Verification items for the finished model (mm, model axes). A direction names the side the tool comes from. Coordinates: 2 decimals unless noted, no trailing zeros. Loops run counter-clockwise (first coordinate to the right, second up) from the corner with the lowest first, then second, coordinate; pieces in that order, holes last.
Q1. Access from +Z, -Z, +X, -X, +Y, -Y to the whole of each face (thin tool, end or side, straight path). Record for faces 1 (the face through (-7.493, 0.33, 29.249)), 2 (the face through (37.497, -16.228, 22.283)), 3 (the face through (-1.409, -17.325, 10.295)).
Q2. Sectioned sample at A-A (x = 0). Enter the section's corners in (y, z), then the cut area to 3 significant figures.
Q3. Sectioned sample at B-B (z = 20.5). Enter the section's corners in (x, y).
Q4. Sectioned sample at C-C (x = 33.5). Enter the section's corners in (y, z), then the cut area to 3 significant figures.
Q5. Material ranges on probe 1 along Y at (x, z) = (-6, 24); probe 2 along Z at (x, y) = (-26.5, -8); probe 3 along Y at (x, z) = (-8, 7.5), recorded low to high.
Q6. Go/stop test with flat-tipped pins: P1, Ø10, axis at x = 9, y = 7, coming from the -Z side; P2, Ø1, axis at y = 9, z = 6, coming from the +X side; P3, Ø12, axis at x = 8.5, y = 1, coming from the -Z side; P4, Ø12, axis at x = -11.5, y = -11, coming from the -Z side. Record where each tip stops, or that it passes through.
```python
from build123d import *

# Parameters (mm, degrees)
BOSS_EXTRUDE1_DEPTH      = 27.77
FILLET1_START            = -44
FILLET1_DEPTH            = 88
FILLET2_R                = 3
SKETCH3_R                = 7.5
BOSS_EXTRUDE2_DEPTH      = 3
BOSS_EXTRUDE3_DEPTH      = 2
BOSS_EXTRUDE3_DEPTH_BACK = 3
SKETCH4_R                = 6.5


with BuildPart() as part:
    # Sketch2 → Boss-Extrude1 (new body)
    with BuildSketch(Plane.XY):
        with BuildLine():
            Line((-37.65, 16.64), (37.65, 16.64))
            ThreePointArc((37.65, 16.64), (42.65, 0), (37.65, -16.64))
            Line((37.65, -16.64), (-37.65, -16.64))
            ThreePointArc((-37.65, -16.64), (-42.65, 0), (-37.65, 16.64))
        make_face()
    extrude(amount=BOSS_EXTRUDE1_DEPTH)

    # Fillet1: read off the stored shape, not the designer's step
    # Fillet1 outline → Fillet1 (cut)
    with BuildSketch(Plane.YZ.offset(FILLET1_START)):
        with BuildLine():
            Line((16.64, 0), (16.64, 16.64))
            ThreePointArc((16.64, 16.64), (11.766256851, 4.873743173), (3.4e-08, 0))
            Line((3.4e-08, 0), (16.64, 0))
        make_face()
        with BuildLine():
            Line((-16.64, 0), (3.4e-08, 0))
            ThreePointArc((3.4e-08, 0), (-11.766256827, 4.873743149), (-16.64, 16.64))
            Line((-16.64, 16.64), (-16.64, 0))
        make_face()
    extrude(amount=FILLET1_DEPTH, mode=Mode.SUBTRACT)

    # Fillet2
    fillet2_edges = [part.edges().sort_by_distance(p)[0] for p in [
        (40.256336976, -11.781119236, 4.888624385),
        (-40.256337033, -11.781119103, 4.888624252),
        (-37.65, 16.64, 22.205),
        (37.65, 16.64, 22.205),
        (37.65, -16.64, 22.205),
        (-37.65, -16.64, 22.205),
    ]]
    fillet(fillet2_edges, radius=FILLET2_R)

    # Sketch3 → Boss-Extrude2 (add)
    with BuildSketch(Plane.XY.offset(27.77)):
        Circle(SKETCH3_R)
    extrude(amount=BOSS_EXTRUDE2_DEPTH)

    # Sketch4 → Boss-Extrude3 (add, two sides: drawn at the far end of the back side and taken through both)
    with BuildSketch(Plane.XZ.offset(16.64).offset(-BOSS_EXTRUDE3_DEPTH_BACK)):
        with Locations((0, 16.64)):
            Circle(SKETCH4_R)
    extrude(amount=BOSS_EXTRUDE3_DEPTH + BOSS_EXTRUDE3_DEPTH_BACK)


solid = part.part
```
Geometry check:
1. face 1: +Z
1. face 2: +Z, -Z, +X, -Y
1. face 3: -Y
2. outline: (-18.64, 10.14) - (-15.32, 10.14) arc R16.64 ccw to (16.64, 16.64) - (16.64, 27.77) - (7.5, 27.77) - (7.5, 30.77) - (-7.5, 30.77) - (-7.5, 27.77) - (-16.64, 27.77) - (-16.64, 23.14) - (-18.64, 23.14) - close
2. area: 879 mm2
3. outline: (-38.58, -15.15) arc R3 ccw to (-35.98, -16.64) - (-5.23, -16.64) - (-5.23, -18.64) - (5.23, -18.64) - (5.23, -16.64) - (35.98, -16.64) arc R3 ccw to (38.58, -15.15) arc R30.19 ccw to (38.58, 15.15) arc R3 ccw to (35.98, 16.64) - (-35.98, 16.64) arc R3 ccw to (-38.58, 15.15) arc R30.19 ccw to start
4. outline: (-16.64, 16.64) arc R16.64 ccw to (16.64, 16.64) - (16.64, 27.77) - (-16.64, 27.77) - close
4. area: 805 mm2
5. probe 1: y = -16.64 to 16.64
5. probe 2: z = 2.05 to 27.77
5. probe 3: y = -13.91 to 13.91
6. P1: stops at z = 0.12
6. P2: stops at x = 41.43
6. P3: stops at z = 0
6. P4: stops at z = 0.77
